Geometry check sheet. Reference: drawing and pictorial views, mm from the part's lowest x, y, z. A direction names the side the tool comes from. Give positions to 0.01 mm unless a question says otherwise; leave off trailing zeros. Order: outer loops, then holes, each group sorted by start corner. A loop starts at its lowest first (then second) coordinate and runs counter-clockwise, first axis right, second up. Notation, with made-up numbers: (-31, 27) - (-2, 27) arc R31 cw to (-2, 55) - close; hole circle Ø7 at (69.5, -29). An arc over 180 degrees is marked (long way). Answer as a JSON object with one key per item and string values.
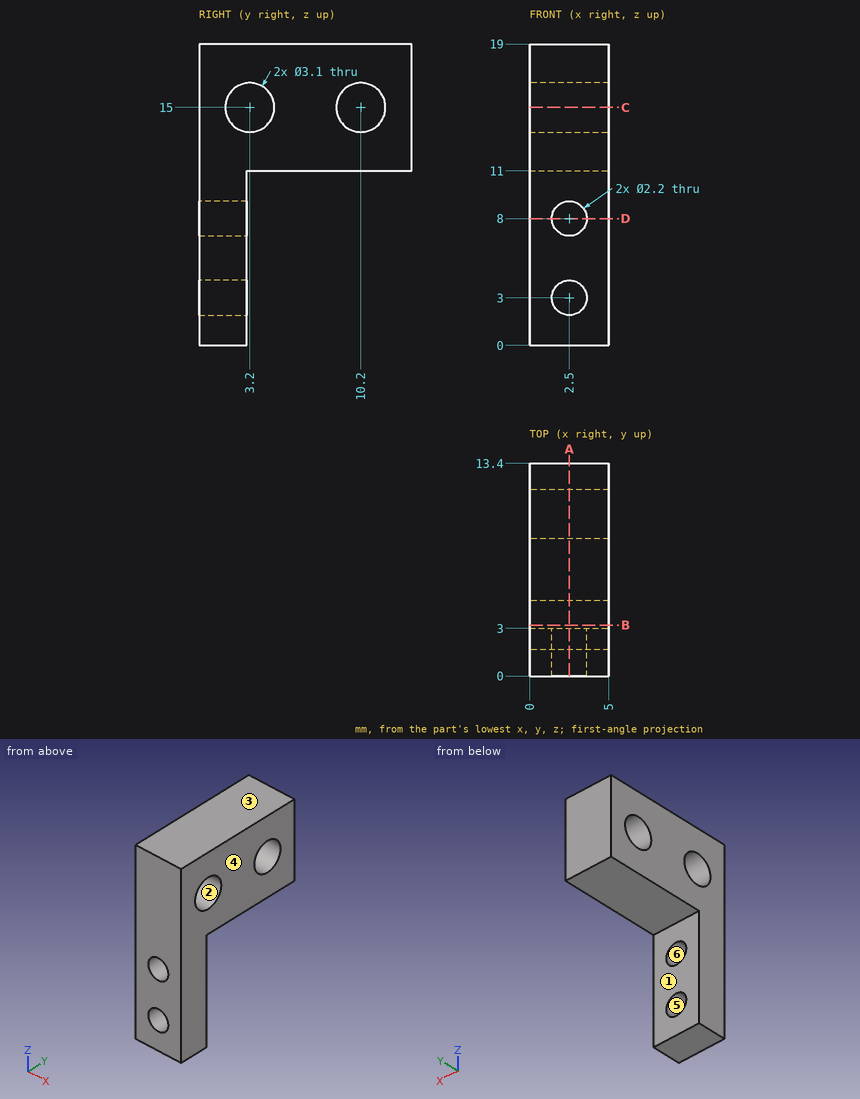
(1) Section check C-C (z = 15). Record the cut outline in (x, y), then the cut area to 3 significant figures.
Computed values:
{"outline": "(0, 0) - (5, 0) - (5, 1.65) - (0, 1.65) - close; (0, 4.75) - (5, 4.75) - (5, 8.65) - (0, 8.65) - close; (0, 11.75) - (5, 11.75) - (5, 13.4) - (0, 13.4) - close", "area": "36.0 mm²"}
(2) Section check D-D (z = 8). Record the cut outline in (x, y), then the cut area to 3 significant figures.
Computed values:
{"outline": "(0, 0) - (1.4, 0) - (1.4, 3) - (0, 3) - close; (3.6, 0) - (5, 0) - (5, 3) - (3.6, 3) - close", "area": "8.40 mm²"}
(3) Material ranges on line 1 along Y through (x, z) = (2.25, 15); line 2 along X through (y, z) = (1.85, 3); line 3 along Z through (x, y) = (3.1, 5), recorded low to high. Write a range as [from, to].
Computed values:
{"line 1": "y = [0, 1.65], [4.75, 8.65], [11.75, 13.4]", "line 2": "x = [0, 1.4], [3.6, 5]", "line 3": "z = [11, 19]"}
(4) Section check B-B (y = 3.2). Record the cut outline in (x, z).
Computed values:
{"outline": "(0, 11) - (5, 11) - (5, 13.45) - (0, 13.45) - close; (0, 16.55) - (5, 16.55) - (5, 19) - (0, 19) - close"}
(5) Access from +Z, -Z, +X, -X, +Y, -Y to the whole of each face (thin tool, end or side, straight path). Record for the marked faces 1 and 2.
Computed values:
{"face 1": "-Z, +X, -X, +Y", "face 2": "+X, -X"}
(6) Release check for a two-part mould opening along X. For the marked faces 3, 4, 5 and 6 record: pulls with the +X half, pulls with the -X half, needs draft (parallel to the pull), parting line crosses it, or undercut.
Computed values:
{"face 3": "needs draft", "face 4": "pulls with the +X half", "face 5": "undercut", "face 6": "undercut"}
(7) Section check A-A (x = 2.5). Record the cut outline in (y, z).
Computed values:
{"outline": "(0, 0) - (3, 0) - (3, 1.9) - (0, 1.9) - close; (0, 4.1) - (3, 4.1) - (3, 6.9) - (0, 6.9) - close; (0, 9.1) - (3, 9.1) - (3, 11) - (13.4, 11) - (13.4, 19) - (0, 19) - close; hole circle Ø3.1 at (3.2, 15); hole circle Ø3.1 at (10.2, 15)"}
(8) Gauge pin test, flat ends, axial feed: pin 1 Ø2 at (x, z) = (0.5, 8) entering from -Y; pin 2 Ø1.5 at (x, y) = (3.5, 5) entering from -Z; pin 3 Ø1.5 at (x, z) = (1.5, 6) entering from +Y. Record the tip position at first contact, or that the pin passes through.
Computed values:
{"pin 1": "stops at y = 0", "pin 2": "stops at z = 11", "pin 3": "stops at y = 3"}
